For this review, take the finished solid that the model builds, in its own axes (mm). Face numbers are marked on the shaded views. Coordinates: 2 decimals unless noted, no trailing zeros. Order: outer loops, then holes, each group sorted by start corner. A loop starts at its lowest first (then second) coordinate and runs counter-clockwise, first axis right, second up. Notation, with made-up numbers: (32.25, -7.5) -> (69.25, -7.5) arc R29 ccw to (69.25, 31.5) -> close; hole circle Ø7 at (11, 85.25). An arc over 180 degrees is marked (long way). Answer as a JSON object with one key per item and string values. Group by question number.
1) Draft analysis for pull direction Y (two halves, no side actions). For the marked faces 1, 2, 3 and 4, state which applies: +Y half, -Y half, draft (parallel to the pull), parting line (faces both ways), or undercut.
2) Add section C-C, the plane x = 0. Write out the cut boundary in (y, z).
3) Add section D-D, the plane x = -5.5. Write out the cut boundary in (y, z).
4) Add section B-B, the plane z = -3.75. Write out the cut boundary in (x, y).
5) Add section A-A, the plane y = 0. Write out the cut boundary in (x, z).
6) Wall thickness on L1, parallel to Y at x = 0, z = -2.75; L2, parallel to Y at x = -4, z = -2.75; L3, parallel to X at y = -1.75, z = 0.5: over which ranges is each line inside the solid? List them lowest first.
7) For pin 1 (12.5 mm diameter, centred on x = 0, y = 0, fed in from +Z), flat-tipped, find the tip position at first contact; note if it passes through.
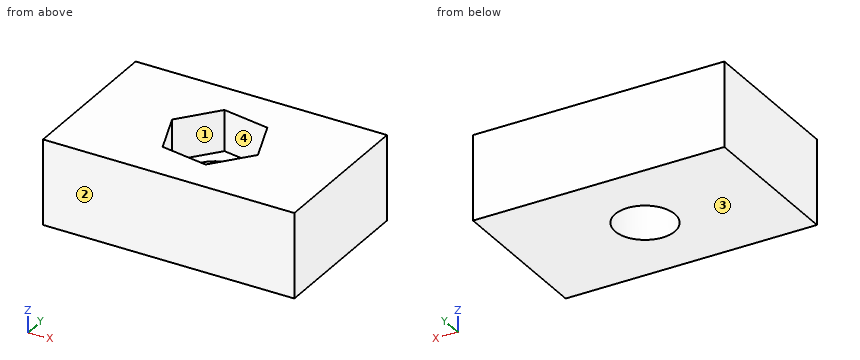
from build123d import *

# Parameters (mm, degrees)
F0_W     = 40
F0_H     = 25
F1_DEPTH = 7
F3_DEPTH = 6.5
F4_R     = 4.75
F5_DEPTH = 10


# Not quite as in the source:
# - a feature names something its author has since deleted; it is built from what else it names


with BuildPart() as f1:
    # F0 (on Top) → F1 (new body)
    with BuildSketch(Plane.XY):
        Rectangle(F0_W, F0_H)
        Polygon((-2.7157951384, 7.1515935357), (4.8355641102, 5.9277443492), (7.5513592486, -1.2238491865), (2.7157951384, -7.1515935357), (-4.8355641102, -5.9277443492), (-7.5513592486, 1.2238491865), align=None, mode=Mode.SUBTRACT)
        Polygon((7.5513592486, -1.2238491865), (4.8355641102, 5.9277443492), (-2.7157951384, 7.1515935357), (-7.5513592486, 1.2238491865), (-4.8355641102, -5.9277443492), (2.7157951384, -7.1515935357), align=None)
    extrude(amount=-F1_DEPTH)

    # F0 (on Top) → F3 (join)
    with BuildSketch(Plane.XY):
        Rectangle(F0_W, F0_H)
        Polygon((-2.7157951384, 7.1515935357), (4.8355641102, 5.9277443492), (7.5513592486, -1.2238491865), (2.7157951384, -7.1515935357), (-4.8355641102, -5.9277443492), (-7.5513592486, 1.2238491865), align=None, mode=Mode.SUBTRACT)
    extrude(amount=F3_DEPTH)

    # F4 (on Top) → F5 (cut)
    with BuildSketch(Plane.XY):
        Circle(F4_R)
    extrude(amount=-F5_DEPTH, mode=Mode.SUBTRACT)


solid = f1.part
Output values:
{
 "1": {"face 1": "undercut", "face 2": "-Y half", "face 3": "draft", "face 4": "undercut"},
 "2": {"outline": "(-12.5, -7) -> (-4.75, -7) -> (-4.75, 0) -> (-6.71, 0) -> (-6.71, 6.5) -> (-12.5, 6.5) -> close; (4.75, -7) -> (12.5, -7) -> (12.5, 6.5) -> (6.71, 6.5) -> (6.71, 0) -> (4.75, 0) -> close"},
 "3": {"outline": "(-12.5, -7) -> (12.5, -7) -> (12.5, 6.5) -> (3.74, 6.5) -> (3.74, 0) -> (-4.18, 0) -> (-4.18, 6.5) -> (-12.5, 6.5) -> close"},
 "4": {"outline": "(-20, -12.5) -> (20, -12.5) -> (20, 12.5) -> (-20, 12.5) -> close; hole circle Ø9.5 at (0, 0)"},
 "5": {"outline": "(-20, -7) -> (-4.75, -7) -> (-4.75, 0) -> (-7.09, 0) -> (-7.09, 6.5) -> (-20, 6.5) -> close; (4.75, -7) -> (20, -7) -> (20, 6.5) -> (7.09, 6.5) -> (7.09, 0) -> (4.75, 0) -> close"},
 "6": {"L1": "y = -12.5 to -4.75, 4.75 to 12.5", "L2": "y = -12.5 to -2.56, 2.56 to 12.5", "L3": "x = -20 to -6.42, 7.12 to 20"},
 "7": {"pin 1": "stops at z = 0"}
}
